Design review of the part built by this model. Coordinates are the model's own, in mm. Face numbers are marked on the shaded views. A direction names the side the tool comes from. Round coordinates to 2 decimals unless told otherwise and drop trailing zeros. Write each loop counter-clockwise with the first axis right and the second up, starting at its lowest first coordinate (ties: lowest second). Pieces come first, ordered by that corner, then holes. Notation, with made-up numbers: M -18,73.25 L -14,73.25 A15 cw -14,77.25 Z; hole C 11.5,-7.75 d1. An arc over 180 degrees is marked long. One line per question, with ' | ' between items. Start each with the question number.
Item 1: Add section A-A, the plane x = 42.5. State the section outline as (y, z) points, and give its area (3 significant figures).
Item 2: Insertion check: pin 1 Ø6 at (x, z) = (10.42, -12.5) entering from -Y; pin 2 Ø5 at (x, z) = (60, -17.5) entering from +Y; pin 3 Ø12 at (y, z) = (26.5, -18.5) entering from +X; pin 4 Ø1 at (y, z) = (19, -17) entering from -X. Each pin has a flat end and moves straight along its axis. Give the tip position at first contact, or say it passes through.
Item 3: Add section B-B, the plane y = 4.5. State the section outline as (x, z) points, and give its area (3 significant figures).
Item 4: Machinability: for the marked faces 4, 5 and 6, which of the approach directions +Z, -Z, +X, -X, +Y, -Y give a long, thin tool a straight path to every point of the face, cutting with its end or side? Answer none if there is none.
Item 5: Draft analysis for pull direction Z (two halves, no side actions). For the marked faces 1, 2 and 3, state which applies: released by +Z, released by -Z, zero draft, split by the parting line, or undercut.
Item 6: Add section C-C, the plane z = -12.5. State the section outline as (x, y) points, and give its area (3 significant figures).
Item 7: Add section D-D, the plane z = -23. State the section outline as (x, y) points.
Item 8: For L1, parallel to X at y = 5.5, z = -12.5; L2, parallel to Z at x = 10.5, y = 1.5; L3, parallel to Y at x = 50.5, z = -4.5, list the stretches that pass through material, from the lowest coordinate up.
```python
from build123d import *

# Parameters (mm, degrees)
SKETCH2_W                                           = 85
SKETCH2_H                                           = 25
BOSS_EXTRUDE1_DEPTH                                 = 15
BOSS_EXTRUDE3_DEPTH                                 = 25
CSK_FOR_1_4_FLAT_HEAD_MACHINE_SCREW_100_D           = 6.7564
CSK_FOR_1_4_FLAT_HEAD_MACHINE_SCREW_100_CSINK_D     = 12.8778
CSK_FOR_1_4_FLAT_HEAD_MACHINE_SCREW_100_CSINK_ANGLE = 100
SKETCH7_W                                           = 21.650635094
SKETCH7_H                                           = 3.75
CUT_EXTRUDE1_DEPTH                                  = 55


with BuildPart() as part:
    # Sketch2 → Boss-Extrude1 (new body)
    with BuildSketch(Plane(origin=(0, 0, 0), x_dir=(1, 0, 0), z_dir=(0, 1, 0))):
        with Locations((42.5, 12.5)):
            Rectangle(SKETCH2_W, SKETCH2_H)
    extrude(amount=BOSS_EXTRUDE1_DEPTH)

    # Sketch6 → Boss-Extrude3 (add)
    with BuildSketch(Plane.XY):
        with BuildLine():
            Line((20.849364905, 15), (64.150635095, 15))
            ThreePointArc((64.150635095, 15), (42.5, 30.412878475), (20.849364905, 15))
        make_face()
    extrude(amount=-BOSS_EXTRUDE3_DEPTH)

    # CSK for 1_4 Flat Head Machine Screw _100 (through all)
    with Locations(Plane(origin=(0, 15, 0), x_dir=(1, 0, 0), z_dir=(0, 1, 0))):
        with Locations((74.575317547, 12.5), (10.424682453, 12.5)):
            CounterSinkHole(CSK_FOR_1_4_FLAT_HEAD_MACHINE_SCREW_100_D / 2, CSK_FOR_1_4_FLAT_HEAD_MACHINE_SCREW_100_CSINK_D / 2, counter_sink_angle=CSK_FOR_1_4_FLAT_HEAD_MACHINE_SCREW_100_CSINK_ANGLE)

    # Sketch7 → Cut-Extrude1 (cut)
    with BuildSketch(Plane.XY):
        with BuildLine():
            Line((34.781122165, 7.5), (50.218877835, 7.5))
            ThreePointArc((50.218877835, 7.5), (42.5, 25.762484612), (34.781122165, 7.5))
        make_face()
        with BuildLine():
            ThreePointArc((36.168863864, 6.296679355), (48.955812715, 23.611245974), (35.920849566, 6.482614569))
            Line((35.920849566, 6.482614569), (36.168863864, 6.296679355))
        make_face()
        with Locations((42.5, 5.625)):
            Rectangle(SKETCH7_W, SKETCH7_H)
        with BuildLine():
            ThreePointArc((36.168863864, 6.296679355), (43.418396374, 4.276771796), (50.218877835, 7.5))
            Line((50.218877835, 7.5), (34.781122165, 7.5))
            ThreePointArc((34.781122165, 7.5), (35.332910537, 6.971058373), (35.920849566, 6.482614569))
            Line((35.920849566, 6.482614569), (36.168863864, 6.296679355))
        make_face()
    extrude(amount=-CUT_EXTRUDE1_DEPTH, mode=Mode.SUBTRACT)


solid = part.part
```
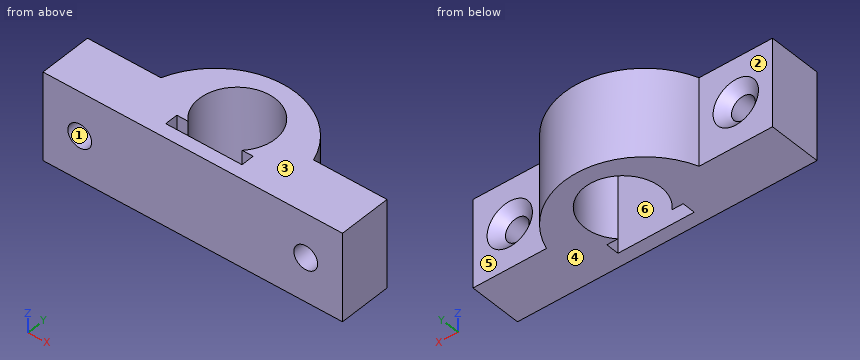
Computed values:
1) outline: M 0,-25 L 3.75,-25 L 3.75,0 L 0,0 Z; M 25.76,-25 L 30.41,-25 L 30.41,0 L 25.76,0 Z | area: 210 mm^2
2) pin 1: passes through | pin 2: stops at y = 24.82 | pin 3: stops at x = 61.37 | pin 4: stops at x = 22.4
3) outline: M 0,-25 L 31.67,-25 L 31.67,0 L 0,0 Z; M 53.33,-25 L 85,-25 L 85,0 L 53.33,0 Z; hole C 10.42,-12.5 d6.76; hole C 74.58,-12.5 d6.76 | area: 1,510 mm^2
4) face 4: -Z, +X, -X, +Y, -Y | face 5: +Z, -Z, +X, +Y | face 6: +Z, -Z
5) face 1: undercut | face 2: zero draft | face 3: released by +Z
6) outline: M 0,0 L 7.05,0 L 7.05,12.43 L 3.99,15 L 0,15 Z; M 13.8,0 L 71.2,0 L 71.2,12.43 L 68.14,15 L 64.15,15 A22.91 ccw 20.85,15 L 16.86,15 L 13.8,12.43 Z; M 77.95,0 L 85,0 L 85,15 L 81.01,15 L 77.95,12.43 Z; hole M 31.67,3.75 L 53.33,3.75 L 53.33,7.5 L 50.22,7.5 A10.76 ccw long 34.78,7.5 L 31.67,7.5 Z | area: 1,130 mm^2
7) outline: M 0,0 L 85,0 L 85,15 L 64.15,15 A22.91 ccw 20.85,15 L 0,15 Z; hole M 31.67,3.75 L 53.33,3.75 L 53.33,7.5 L 50.22,7.5 A10.76 ccw long 34.78,7.5 L 31.67,7.5 Z
8) L1: x = 0 to 7.05, 13.8 to 31.67, 53.33 to 71.2, 77.95 to 85 | L2: z = -25 to -15.88, -9.12 to 0 | L3: y = 0 to 3.75, 7.5 to 7.8, 22.2 to 28.97
